Could you check a few things on this model? Use its own coordinates, in mm. A direction names the side the tool comes from. Give positions to 0.01 mm unless a question says otherwise; leave off trailing zeros. Loops run counter-clockwise (first coordinate to the right, second up) from the corner with the lowest first, then second, coordinate; pieces in that order, holes last. Notation, with made-up numbers: (85.25, 82.25) - (128.25, 82.25) arc R14 cw to (128.25, 92.25) - close; hole circle Ø3 at (78.25, 52). An arc over 180 degrees is marked (long way). Write each question's results on one line, items separated by ' | '. Start each with the question number.
(1) Suppose I cut it at B-B (z = -6.5). Please give me the cut outline in (x, y), and give its area (3 significant figures).
(2) Suppose I cut it at C-C (y = -1.55). Count the separate pieces of the cut face and the enclosed holes in it, and give its area (3 significant figures).
(3) I need wall thicknesses on line 1 (X direction, y = -2.9, z = -108); line 2 (X direction, y = -2.55, z = -41); line 3 (X direction, y = -2.7, z = -40.5). Which ranges of each line are inside material? Lowest first, please.
(4) If we mould it in two halves opening along X, with no side actions, what happens to faces 3 (the face through (59, -2, -43)), 4 (the face through (59, -2, -120))? For each: released by +X, released by -X, zero draft, split by the parting line, or undercut.
(5) On a 3-axis mill with a long thin cutter (end or side, diameter ignored), from which of +Z, -Z, +X, -X, +Y, -Y can I reach the whole of each face in a straight line? I mean faces 1 (the face through (59, -2, 0)), 2 (the face through (59, -2, -71)). Say none if no direction works.
(6) Suppose I cut it at A-A (x = 6.5). Please give me the cut outline in (y, z).
from build123d import *

# Parameters (mm, degrees)
SKETCH1_W           = 120
SKETCH1_H           = 120
SKETCH1_R           = 3
SKETCH1_W_2         = 100
SKETCH1_H_2         = 3
BOSS_EXTRUDE1_DEPTH = 4
FILLET1_R           = 1
FILLET2_R           = 1


with BuildPart() as part:
    # Sketch1 → Boss-Extrude1 (new body)
    with BuildSketch(Plane(origin=(0, 0, 0), x_dir=(1, 0, 0), z_dir=(0, 1, 0))):
        with Locations((60, 60)):
            Rectangle(SKETCH1_W, SKETCH1_H)
        with Locations(Location((113.5, 6.5, 0), (0, 0, 270))):
            Circle(SKETCH1_R, mode=Mode.SUBTRACT)
        with Locations(Location((6.5, 6.5, 0), (0, 0, 270))):
            Circle(SKETCH1_R, mode=Mode.SUBTRACT)
        with Locations(Location((113.5, 108, 0), (0, 0, 270))):
            Circle(SKETCH1_R, mode=Mode.SUBTRACT)
        with Locations(Location((6.5, 108, 0), (0, 0, 270))):
            Circle(SKETCH1_R, mode=Mode.SUBTRACT)
        with Locations((60, 13.5)):
            Rectangle(SKETCH1_W_2, SKETCH1_H_2, mode=Mode.SUBTRACT)
        with Locations((60, 69.5)):
            Rectangle(SKETCH1_W_2, SKETCH1_H_2, mode=Mode.SUBTRACT)
        with Locations((60, 26.5)):
            Rectangle(SKETCH1_W_2, SKETCH1_H_2, mode=Mode.SUBTRACT)
        with Locations((60, 41.5)):
            Rectangle(SKETCH1_W_2, SKETCH1_H_2, mode=Mode.SUBTRACT)
        with Locations((60, 56.5)):
            Rectangle(SKETCH1_W_2, SKETCH1_H_2, mode=Mode.SUBTRACT)
        with Locations((60, 85.5)):
            Rectangle(SKETCH1_W_2, SKETCH1_H_2, mode=Mode.SUBTRACT)
        with Locations((60, 100.5)):
            Rectangle(SKETCH1_W_2, SKETCH1_H_2, mode=Mode.SUBTRACT)
        with Locations((60, 115.5)):
            Rectangle(SKETCH1_W_2, SKETCH1_H_2, mode=Mode.SUBTRACT)
    extrude(amount=-BOSS_EXTRUDE1_DEPTH)

    # Fillet1
    fillet1_edges = [part.edges().sort_by_distance(p)[0] for p in [
        (110, -2, -15),
        (10, -2, -15),
        (10, -2, -12),
        (110, -2, -12),
        (110, -2, -28),
        (10, -2, -28),
        (10, -2, -25),
        (110, -2, -25),
        (110, -2, -43),
        (10, -2, -43),
        (10, -2, -40),
        (110, -2, -40),
        (110, -2, -58),
        (10, -2, -58),
        (10, -2, -55),
        (110, -2, -55),
        (110, -2, -71),
        (10, -2, -71),
        (10, -2, -68),
        (110, -2, -68),
        (110, -2, -87),
        (10, -2, -87),
        (10, -2, -84),
        (110, -2, -84),
        (110, -2, -102),
        (10, -2, -102),
        (10, -2, -99),
        (110, -2, -99),
        (110, -2, -117),
        (10, -2, -117),
        (10, -2, -114),
        (110, -2, -114),
    ]]
    fillet(fillet1_edges, radius=FILLET1_R)

    # Fillet2
    fillet2_edges = [part.edges().sort_by_distance(p)[0] for p in [
        (0, -2, 0),
        (0, -2, -120),
        (120, -2, -120),
        (120, -2, 0),
    ]]
    fillet(fillet2_edges, radius=FILLET2_R)


solid = part.part
Output values:
1) outline: (0, -4) - (3.5, -4) - (3.5, 0) - (0, 0) - close; (9.5, -4) - (110.5, -4) - (110.5, 0) - (9.5, 0) - close; (116.5, -4) - (120, -4) - (120, 0) - (116.5, 0) - close | area: 432 mm2
2) separate pieces: 1 | enclosed holes: 12 | area: 11,900 mm2
3) line 1: 0 to 3.5, 9.5 to 110.5, 116.5 to 120 | line 2: 0 to 10, 110 to 120 | line 3: 0 to 10.13, 109.87 to 120
4) face 3: undercut | face 4: zero draft
5) face 1: +Z, +X, -X, +Y, -Y | face 2: +Y, -Y
6) outline: (-4, -120) - (0, -120) - (0, -111) - (-4, -111) - close; (-4, -105) - (0, -105) - (0, -9.5) - (-4, -9.5) - close; (-4, -3.5) - (0, -3.5) - (0, 0) - (-4, 0) - close
